Verification items for this drawing (mm, ordinates from the low corner). A direction names the side the tool comes from. Coordinates: 2 decimals unless noted, no trailing zeros. Order: outer loops, then holes, each group sorted by start corner. A loop starts at its lowest first (then second) coordinate and runs counter-clockwise, first axis right, second up. Notation, with made-up numbers: M 6,56 L 45,56 A28 cw 45,91 Z; hole C -17.5,38.5 d11. An arc over 180 degrees is marked long. Answer as a JSON object with one key per item and string values. Group by question number.
(1) Mould release check, pull along X, two halves, no side actions. Record for the marked faces 3, 4 and 5: released by +X, released by -X, zero draft, split by the parting line, or undercut.
(2) Cross-section at B-B (z = 50.5). Enter the section's corners in (x, y).
(3) Cross-section at A-A (x = 30). Enter the section's corners in (y, z).
(4) Access from +Z, -Z, +X, -X, +Y, -Y to the whole of each face (thin tool, end or side, straight path). Record for the marked faces 1 and 2.
(5) Gauge pin test, flat end, axial feed: pin 1 Ø0.5 at (x, y) = (35.5, 0.5) entering from +Z. Record the tip position at first contact, or that the pin passes through.
(6) Material ranges on line 1 (X direction, y = 55, z = 22.5), recorded low to high.
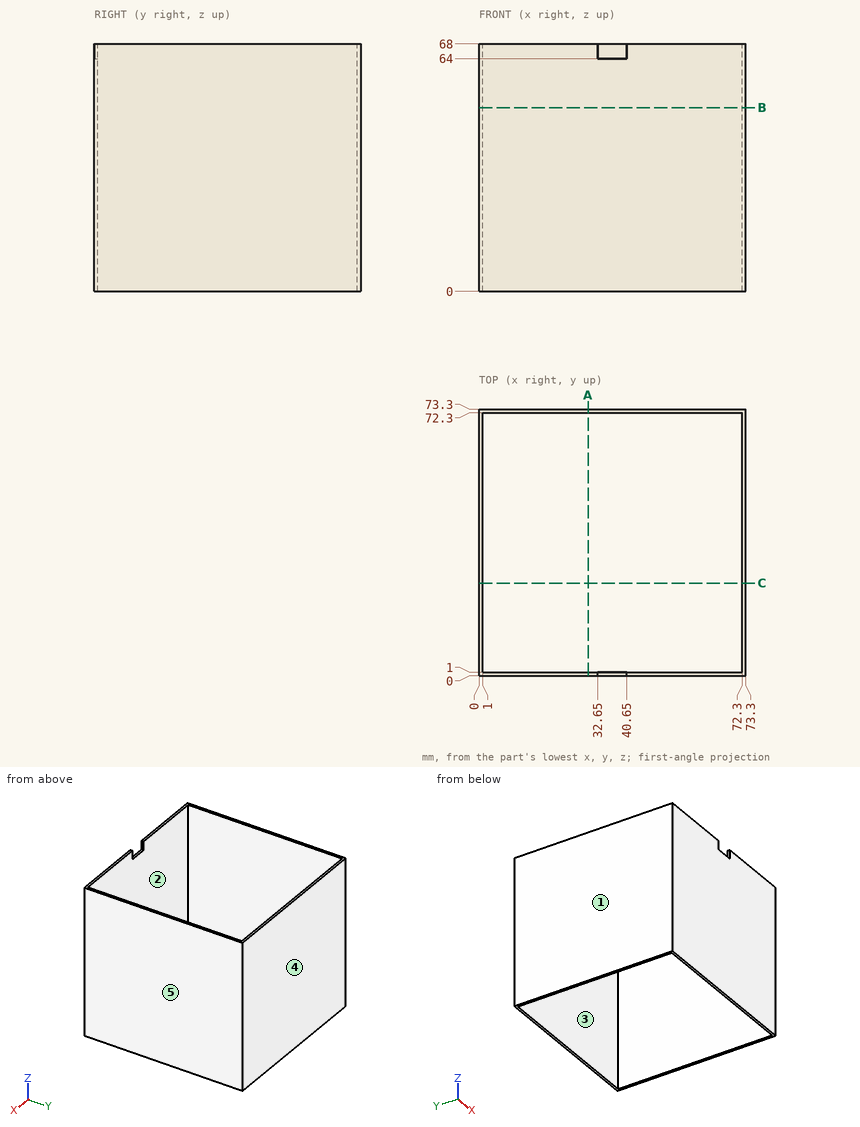
Taken from the geometry:
{
 "1": {"face 3": "undercut", "face 4": "zero draft", "face 5": "released by +X"},
 "2": {"outline": "M 0,0 L 73.3,0 L 73.3,73.3 L 0,73.3 Z; hole M 1,1 L 72.3,1 L 72.3,72.3 L 1,72.3 Z"},
 "3": {"outline": "M 0,0 L 1,0 L 1,68 L 0,68 Z; M 72.3,0 L 73.3,0 L 73.3,68 L 72.3,68 Z"},
 "4": {"face 1": "+Z, -Z, -X, +Y, -Y", "face 2": "+Z, -Z"},
 "5": {"pin 1": "stops at z = 64"},
 "6": {"line 1": "x = 0 to 1, 72.3 to 73.3"}
}
